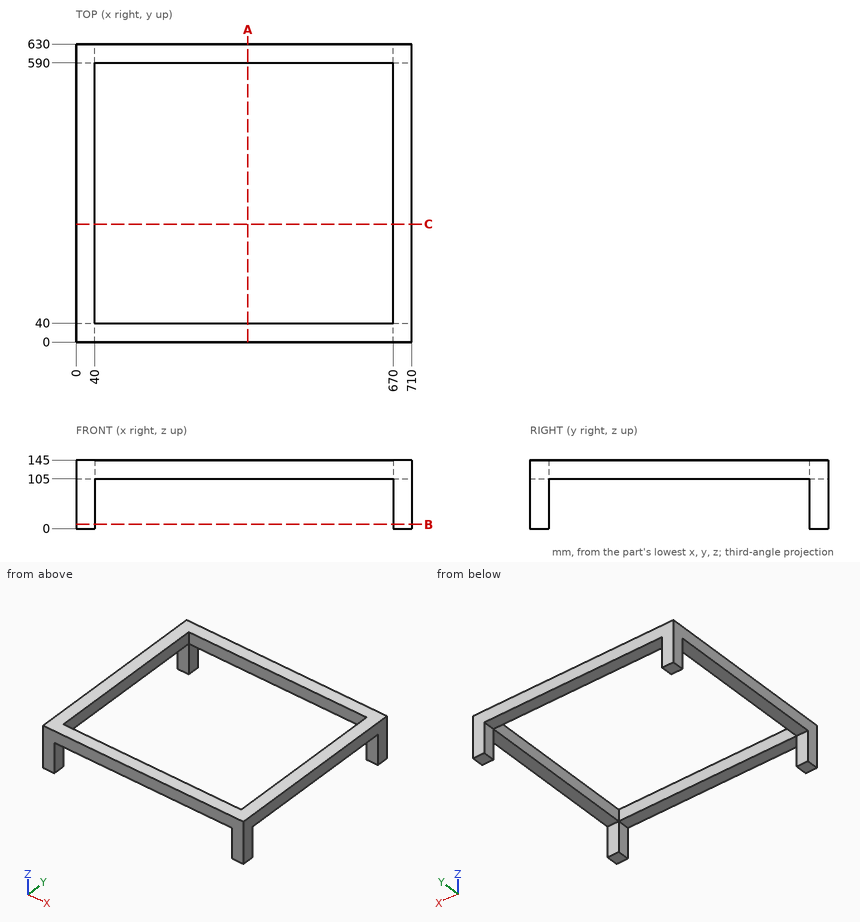
Design review of the part shown in the three views and the two pictorial views. Dimensions are in mm from the part's minimum x, y and z. Coordinates: 2 decimals unless noted, no trailing zeros. Loops run counter-clockwise (first coordinate to the right, second up) from the corner with the lowest first, then second, coordinate; pieces in that order, holes last.
(1) Wall thickness on L1, parallel to Y at x = 45, z = 118; L2, parallel to X at y = 208.5, z = 118; L3, parallel to Z at x = 32.5, y = 444: over which ranges is each line inside the solid? List them lowest first.
Determined:
L1: y = 0 to 40, 590 to 630
L2: x = 0 to 40, 670 to 710
L3: z = 105 to 145
(2) Consider section B-B, the plane z = 9. Give the boundary of the cut face in (x, y).
Determined:
outline: (0, 0) - (40, 0) - (40, 40) - (0, 40) - close; (0, 590) - (40, 590) - (40, 630) - (0, 630) - close; (670, 0) - (710, 0) - (710, 40) - (670, 40) - close; (670, 590) - (710, 590) - (710, 630) - (670, 630) - close
(3) Consider section A-A, the plane x = 363. Give the boundary of the cut face in (y, z).
Determined:
outline: (0, 105) - (40, 105) - (40, 145) - (0, 145) - close; (590, 105) - (630, 105) - (630, 145) - (590, 145) - close
(4) Consider section C-C, the plane y = 249.5. Give the boundary of the cut face in (x, z).
Determined:
outline: (0, 105) - (40, 105) - (40, 145) - (0, 145) - close; (670, 105) - (710, 105) - (710, 145) - (670, 145) - close
(5) Insertion check: P1, Ø20, axis at x = 19, y = 362.5, coming from the -Z side. The pin has a flat end and moves straight along its axis. Give the tip position at first contact, or say it passes through.
Determined:
P1: stops at z = 105
